from build123d import *

# Parameters (mm, degrees)
F0_W     = 97.767125
F0_H     = 12.5
F1_DEPTH = 13.5
F3_DEPTH = 10


with BuildPart() as f1:
    # F0 (on Front) → F1 (new body)
    with BuildSketch(Plane.XZ):
        with Locations((-1.513699, 19.75)):
            Rectangle(F0_W, F0_H)
    extrude(amount=F1_DEPTH)

    # F2 (on Right) → F3 (join)
    with BuildSketch(Plane.YZ):
        with BuildLine():
            ThreePointArc((4.961186, 24.821395), (3.170716, 29.143972), (-1.151862, 30.934442))
            Line((-1.151862, 30.934442), (-12.06661, 30.934442))
            ThreePointArc((-12.06661, 30.934442), (-16.534783, 29.083664), (-18.385561, 24.615491))
            Line((-18.385561, 24.615491), (-18.385561, 13.716214))
            Line((-18.385561, 13.716214), (-13.716212, 13.716214))
            Line((-13.716212, 13.716214), (-13.706157, 13.716214))
            Line((-13.706157, 13.716214), (-13.706157, 26.142228))
            Line((-13.706157, 26.142228), (0, 26.142228))
            Line((0, 26.142228), (0, 13.773428))
            ThreePointArc((0, 13.773428), (3.54785, 15.704206), (4.961186, 19.488069))
            Line((4.961186, 19.488069), (4.961186, 24.821395))
        make_face()
        Polygon((-13.716212, 13.716214), (-18.385561, 13.716214), (-18.385561, 6.858107), (-18.385561, 0), (-13.716212, 0), align=None)
        with BuildLine():
            Line((-18.385561, 0), (-18.385561, 6.858107))
            Line((-18.385561, 6.858107), (-32.718604, 6.858107))
            ThreePointArc((-32.718604, 6.858107), (-35.239143, 5.814066), (-36.283184, 3.293528))
            Line((-36.283184, 3.293528), (-36.283184, 2.944212))
            ThreePointArc((-36.283184, 2.944212), (-35.420844, 0.86234), (-33.338972, 0))
            Line((-33.338972, 0), (-18.385561, 0))
        make_face()
    extrude(amount=F3_DEPTH)


solid = f1.part
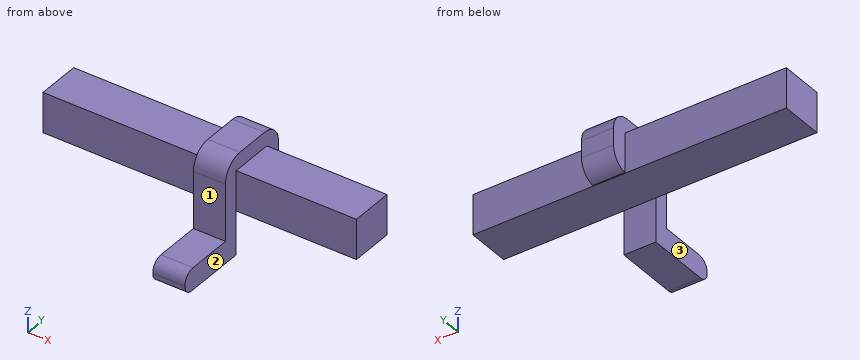
The listing builds one solid part. Answer for the finished solid, in the listing's coordinates (mm). Face numbers are marked on the shaded views. A direction names the side the tool comes from. Give positions to 0.01 mm unless a question says otherwise; leave off trailing zeros. Write each loop counter-clockwise with the first axis right and the second up, starting at its lowest first coordinate (ties: lowest second). Pieces come first, ordered by that corner, then holes.
1) A tool of negligible diameter and unlimited length cuts with its end or side. For the marked faces 1, 2 and 3, from which of +Z, -Z, +X, -X, +Y, -Y can it reach the whole face along a straight path? Write none if from no direction.
2) Find the intervals of material crossed by L1, parallel to Y at x = 3.5, z = 24; L2, parallel to Y at x = 2, z = 19; L3, parallel to Z at x = 40, y = -1.5, in increasing order.
3) Section D-D (y = -21) is taken. Write down the section's boundary in (x, z), and give its area (3 significant figures).
4) Section B-B (z = 15) is taken. Write down the section's boundary in (x, y).
5) Section A-A (y = -7.5) is taken. Write down the section's boundary in (x, z).
6) Section C-C (x = 37) is taken. Write down the section's boundary in (y, z).
7) Given P1, Ø8, axis at x = -28, y = -13.5, coming from the -Z side; P2, Ø1.5, axis at x = 12, z = 18.5, coming from the +Y side; P3, Ø15.5, axis at y = -21, z = 8, coming from the -X side, each flat-ended and moving along its own axis, determine where each tip first touches the part or whether it passes through.
Response:
1. face 1: +Z, +X, -X, -Y
1. face 2: +Z, +X
1. face 3: +Z, -X
2. L1: y = -18.39 to -13.71, -13.5 to 4.96
2. L2: y = -18.39 to -13.71, -13.5 to 4.94
2. L3: z = 13.5 to 26
3. outline: (0, 0) - (10, 0) - (10, 6.86) - (0, 6.86) - close
3. area: 68.6 mm2
4. outline: (-50.4, -13.5) - (47.37, -13.5) - (47.37, 0) - (10, 0) - (10, 2.82) - (0, 2.82) - (0, 0) - (-50.4, 0) - close; (0, -18.39) - (10, -18.39) - (10, -13.71) - (0, -13.71) - close
5. outline: (-50.4, 13.5) - (47.37, 13.5) - (47.37, 26) - (-50.4, 26) - close; (0, 26.14) - (10, 26.14) - (10, 30.93) - (0, 30.93) - close
6. outline: (-13.5, 13.5) - (0, 13.5) - (0, 26) - (-13.5, 26) - close
7. P1: stops at z = 13.5
7. P2: stops at y = 0
7. P3: stops at x = 0
